```python
from build123d import *

# Parameters (mm, degrees)
SKETCH1_R           = 2
BOSS_EXTRUDE1_DEPTH = 3.35
SKETCH2_R           = 3.25
SKETCH2_R_2         = 2
BOSS_EXTRUDE2_DEPTH = 1.75
FILLET1_R           = 1


with BuildPart() as part:
    # Sketch1 → Boss-Extrude1 (new body)
    with BuildSketch(Plane(origin=(0, 0, 0), x_dir=(1, 0, 0), z_dir=(0, 1, 0))):
        Polygon((0, 3.983716857), (-3.45, 1.991858429), (-3.45, -1.991858429), (0, -3.983716857), (3.45, -1.991858429), (3.45, 1.991858429), align=None)
        Circle(SKETCH1_R, mode=Mode.SUBTRACT)
    extrude(amount=BOSS_EXTRUDE1_DEPTH)

    # Sketch2 → Boss-Extrude2 (add)
    with BuildSketch(Plane(origin=(0, 3.35, 0), x_dir=(1, 0, 0), z_dir=(0, 1, 0))):
        Circle(SKETCH2_R)
        Circle(SKETCH2_R_2, mode=Mode.SUBTRACT)
    extrude(amount=BOSS_EXTRUDE2_DEPTH)

    # Fillet1
    fillet1_edges = [part.edges().sort_by_distance(p)[0] for p in [
        (-3.25, 5.1, 0),
    ]]
    fillet(fillet1_edges, radius=FILLET1_R)


solid = part.part
```
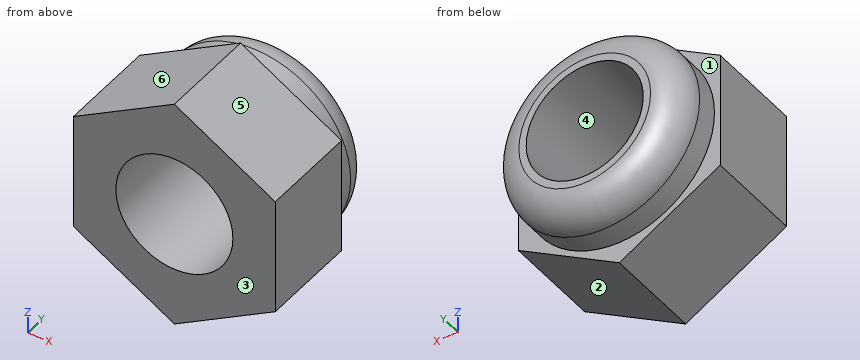
Can you work these out from the model? Positions are in its coordinate system, mm. Face numbers are marked on the shaded views. A direction names the side the tool comes from. Round coordinates to 2 decimals unless told otherwise and drop trailing zeros. Loops run counter-clockwise (first coordinate to the right, second up) from the corner with the lowest first, then second, coordinate; pieces in that order, holes last. Notation, with made-up numbers: M 58,48.5 L 97,48.5 A32 cw 97,83.5 Z; hole C -13.5,-29.75 d5. An arc over 180 degrees is marked long. Answer as a JSON object with one key per item and string values. Group by question number.
Q1. Please list where these lines run through material, in increasing order: L1, parallel to X at y = 3.25, z = 0; L2, parallel to Y at x = 2, z = 2.75; L3, parallel to X at y = 3.55, z = 0.
Q2. Imagine slicing it at A-A, the plane y = 2.2. Please give me the cut outline in (x, z), then the cut area to 3 significant figures.
Q3. Imagine slicing it at B-B, the plane z = 0. Please give me the cut outline in (x, y).
Q4. Will these pins go through, and if not, where does the flat tip stop? pin 1 (1 mm diameter, centred on x = -2, y = 3, fed in from +Z); pin 2 (1 mm diameter, centred on x = -0.5, z = -0.5, fed in from -Y); pin 3 (1 mm diameter, centred on x = 2, y = 1, fed in from -Z); pin 4 (1 mm diameter, centred on y = 4.5, z = 1.5, fed in from -X).
Q5. Imagine slicing it at C-C, the plane y = 4.3. Please give me the cut outline in (x, z).
Q6. We'd pull the mould along X, two halves only. Please class the marked faces 3, 4, 5 and 6: +X half, -X half, draft (parallel to the pull), parting line (faces both ways), or undercut.
Q7. On a 3-axis mill with a long thin cutter (end or side, diameter ignored), from which of +Z, -Z, +X, -X, +Y, -Y can I reach the whole of each face in a straight line? I mean the marked faces 1 and 2. Say none if no direction works.
Findings:
{
 "1": {"L1": "x = -3.45 to -2, 2 to 3.45", "L2": "y = 0 to 3.35", "L3": "x = -3.25 to -2, 2 to 3.25"},
 "2": {"outline": "M -3.45,-1.99 L 0,-3.98 L 3.45,-1.99 L 3.45,1.99 L 0,3.98 L -3.45,1.99 Z; hole C 0,0 d4", "area": "28.7 mm2"},
 "3": {"outline": "M -3.45,0 L -2,0 L -2,5.1 L -2.25,5.1 A1 ccw -3.25,4.1 L -3.25,3.35 L -3.45,3.35 Z; M 2,0 L 3.45,0 L 3.45,3.35 L 3.25,3.35 L 3.25,4.1 A1 ccw 2.25,5.1 L 2,5.1 Z"},
 "4": {"pin 1": "stops at z = 3.12", "pin 2": "passes through", "pin 3": "stops at z = -3.12", "pin 4": "stops at x = -3.06"},
 "5": {"outline": "C 0,0 d6.46; hole C 0,0 d4"},
 "6": {"face 3": "draft", "face 4": "undercut", "face 5": "+X half", "face 6": "-X half"},
 "7": {"face 1": "+Y", "face 2": "-Z, +X, +Y, -Y"}
}
